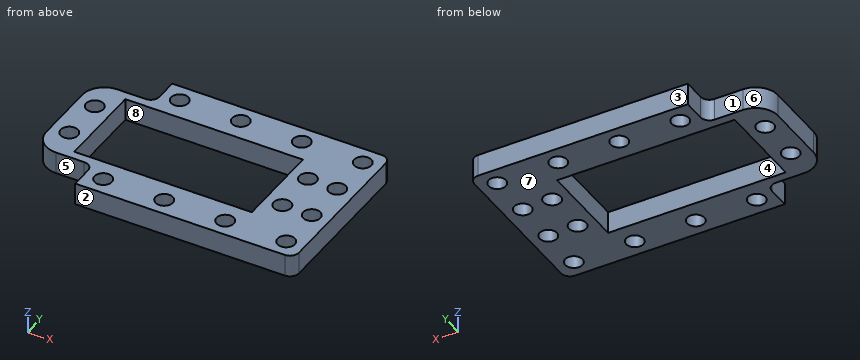
```python
from build123d import *

# Parameters (mm, degrees)
SKETCH1_R           = 1.95
SKETCH1_W           = 40
SKETCH1_H           = 20
BOSS_EXTRUDE1_DEPTH = 5
SKETCH2_W           = 13.39
SKETCH2_H           = 7
CUT_EXTRUDE2_DEPTH  = 6
FILLET1_R           = 2
FILLET2_R           = 5


with BuildPart() as part:
    # Sketch1 → Boss-Extrude1 (new body)
    with BuildSketch(Plane.XY):
        with BuildLine():
            Line((-2, 0), (-60.61, 0))
            ThreePointArc((-60.61, 0), (-62.024213562, -0.585786438), (-62.61, -2))
            Line((-62.61, -2), (-62.61, -36))
            ThreePointArc((-62.61, -36), (-62.024213562, -37.414213562), (-60.61, -38))
            Line((-60.61, -38), (-2, -38))
            ThreePointArc((-2, -38), (-0.585786438, -37.414213562), (0, -36))
            Line((0, -36), (0, -2))
            ThreePointArc((0, -2), (-0.585786438, -0.585786438), (-2, 0))
        make_face()
        with Locations((-10.61, -14)):
            Circle(SKETCH1_R, mode=Mode.SUBTRACT)
        with Locations((-10.61, -24)):
            Circle(SKETCH1_R, mode=Mode.SUBTRACT)
        with Locations((-58.61, -24)):
            Circle(SKETCH1_R, mode=Mode.SUBTRACT)
        with Locations((-58.61, -14)):
            Circle(SKETCH1_R, mode=Mode.SUBTRACT)
        with Locations((-45.22, -4)):
            Circle(SKETCH1_R, mode=Mode.SUBTRACT)
        with Locations((-4, -4)):
            Circle(SKETCH1_R, mode=Mode.SUBTRACT)
        with Locations((-4, -14)):
            Circle(SKETCH1_R, mode=Mode.SUBTRACT)
        with Locations((-58.61, -4)):
            Circle(SKETCH1_R, mode=Mode.SUBTRACT)
        with Locations((-31.48, -4)):
            Circle(SKETCH1_R, mode=Mode.SUBTRACT)
        with Locations((-17.74, -4)):
            Circle(SKETCH1_R, mode=Mode.SUBTRACT)
        with Locations((-45.22, -34)):
            Circle(SKETCH1_R, mode=Mode.SUBTRACT)
        with Locations((-58.61, -34)):
            Circle(SKETCH1_R, mode=Mode.SUBTRACT)
        with Locations((-4, -34)):
            Circle(SKETCH1_R, mode=Mode.SUBTRACT)
        with Locations((-17.74, -34)):
            Circle(SKETCH1_R, mode=Mode.SUBTRACT)
        with Locations((-31.48, -34)):
            Circle(SKETCH1_R, mode=Mode.SUBTRACT)
        with Locations((-4, -24)):
            Circle(SKETCH1_R, mode=Mode.SUBTRACT)
        with Locations((-34.61, -19)):
            Rectangle(SKETCH1_W, SKETCH1_H, mode=Mode.SUBTRACT)
    extrude(amount=BOSS_EXTRUDE1_DEPTH)

    # Sketch2 → Cut-Extrude2 (cut, through all)
    with BuildSketch(Plane.XY.offset(5)):
        with Locations((-55.915, -3.5)):
            Rectangle(SKETCH2_W, SKETCH2_H)
        with Locations((-55.915, -34.5)):
            Rectangle(SKETCH2_W, SKETCH2_H)
    extrude(amount=-CUT_EXTRUDE2_DEPTH, mode=Mode.SUBTRACT)

    # Fillet1
    fillet1_edges = [part.edges().sort_by_distance(p)[0] for p in [
        (-49.22, -7, 2.5),
        (-49.22, -31, 2.5),
    ]]
    fillet(fillet1_edges, radius=FILLET1_R)

    # Fillet2
    fillet2_edges = [part.edges().sort_by_distance(p)[0] for p in [
        (-62.61, -7, 2.5),
        (-62.61, -31, 2.5),
    ]]
    fillet(fillet2_edges, radius=FILLET2_R)


solid = part.part
```
The model under review builds one solid part; all positions refer to its coordinate system, in mm. Face numbers are marked on the shaded views. A direction names the side the tool comes from. Round coordinates to 2 decimals unless told otherwise and drop trailing zeros. Order: outer loops, then holes, each group sorted by start corner. A loop starts at its lowest first (then second) coordinate and runs counter-clockwise, first axis right, second up. Notation, with made-up numbers: M 26.25,-8.75 L 52.25,-8.75 A21 ccw 52.25,26.25 Z; hole C -23,-28.5 d5. An arc over 180 degrees is marked long. Use a Markdown table: item, result.
1) Consider section D-D (x = -10.61). Write out the cut boundary in (y, z), then the cut area to 3 significant figures.
Report:
| item | result |
|---|---|
| outline | M -38,0 L -25.95,0 L -25.95,5 L -38,5 Z; M -22.05,0 L -15.95,0 L -15.95,5 L -22.05,5 Z; M -12.05,0 L 0,0 L 0,5 L -12.05,5 Z |
| area | 151 mm^2 |
2) Consider section C-C (x = -4). Write out the cut boundary in (y, z).
Report:
| item | result |
|---|---|
| outline | M -38,0 L -35.95,0 L -35.95,5 L -38,5 Z; M -32.05,0 L -25.95,0 L -25.95,5 L -32.05,5 Z; M -22.05,0 L -15.95,0 L -15.95,5 L -22.05,5 Z; M -12.05,0 L -5.95,0 L -5.95,5 L -12.05,5 Z; M -2.05,0 L 0,0 L 0,5 L -2.05,5 Z |
3) Tool access review of the marked faces 1, 2, 3, 4 and 5: name each direction out of +Z, -Z, +X, -X, +Y, -Y from which nothing blocks a thin tool from reaching the whole face with its end or side.
Report:
| item | result |
|---|---|
| face 1 | +Z, -Z, -X, +Y |
| face 2 | +Z, -Z, +X, -X, -Y |
| face 3 | +Z, -Z, +X, -X, +Y |
| face 4 | +Z, -Z |
| face 5 | +Z, -Z, -X, -Y |
4) Consider section B-B (z = 3.6). Give the number of separate pieces and of enclosed holes in the cut face, then the cut area to 3 significant figures.
Report:
| item | result |
|---|---|
| separate pieces | 1 |
| enclosed holes | 15 |
| area | 1,210 mm^2 |
5) Consider section A-A (y = -4). Write out the cut boundary in (x, z), then the cut area to 3 significant figures.
Report:
| item | result |
|---|---|
| outline | M -49.22,0 L -47.17,0 L -47.17,5 L -49.22,5 Z; M -43.27,0 L -33.43,0 L -33.43,5 L -43.27,5 Z; M -29.53,0 L -19.69,0 L -19.69,5 L -29.53,5 Z; M -15.79,0 L -5.95,0 L -5.95,5 L -15.79,5 Z; M -2.05,0 L 0,0 L 0,5 L -2.05,5 Z |
| area | 168 mm^2 |
6) Draft analysis for pull direction X (two halves, no side actions). For the marked faces 6, 7 and 8, state which applies: released by +X, released by -X, zero draft, split by the parting line, or undercut.
Report:
| item | result |
|---|---|
| face 6 | released by -X |
| face 7 | zero draft |
| face 8 | undercut |
7) Insertion check: pin 1 (1.5 mm diameter, centred on y = -35, z = 1.5, fed in from -X); pin 2 (1.5 mm diameter, centred on x = -54.5, z = 3.5, fed in from -Y). Each pin has a flat end and moves straight along its axis. Give the tip position at first contact, or say it passes through.
Report:
| item | result |
|---|---|
| pin 1 | x = -49.22 |
| pin 2 | y = -31 |
8) Wall thickness on line 1 along Y through (x, z) = (-4, 2.3); line 2 along Y through (x, z) = (-49, 2.7); line 3 along Y through (x, z) = (-54.5, 4): over which ranges is each line inside the solid? List them lowest first. Write a range as [from, to].
Report:
| item | result |
|---|---|
| line 1 | [-38, -35.95], [-32.05, -25.95], [-22.05, -15.95], [-12.05, -5.95], [-2.05, 0] |
| line 2 | [-38, -29], [-9, 0] |
| line 3 | [-31, -29], [-9, -7] |
